Could you check a few things on this drawing? It's one solid part, dimensions in mm from its lowest x, y, z. Give positions to 0.01 mm unless a question says otherwise; leave off trailing zeros. Loops run counter-clockwise (first coordinate to the right, second up) from the corner with the lowest first, then second, coordinate; pieces in that order, holes last. Notation, with made-up numbers: M -29,69.25 L 10,69.25 A15 cw 10,76.25 Z; hole C 68.5,54 d1. An arc over 180 degrees is marked long. Answer as a JSON object with one key per item and string values.
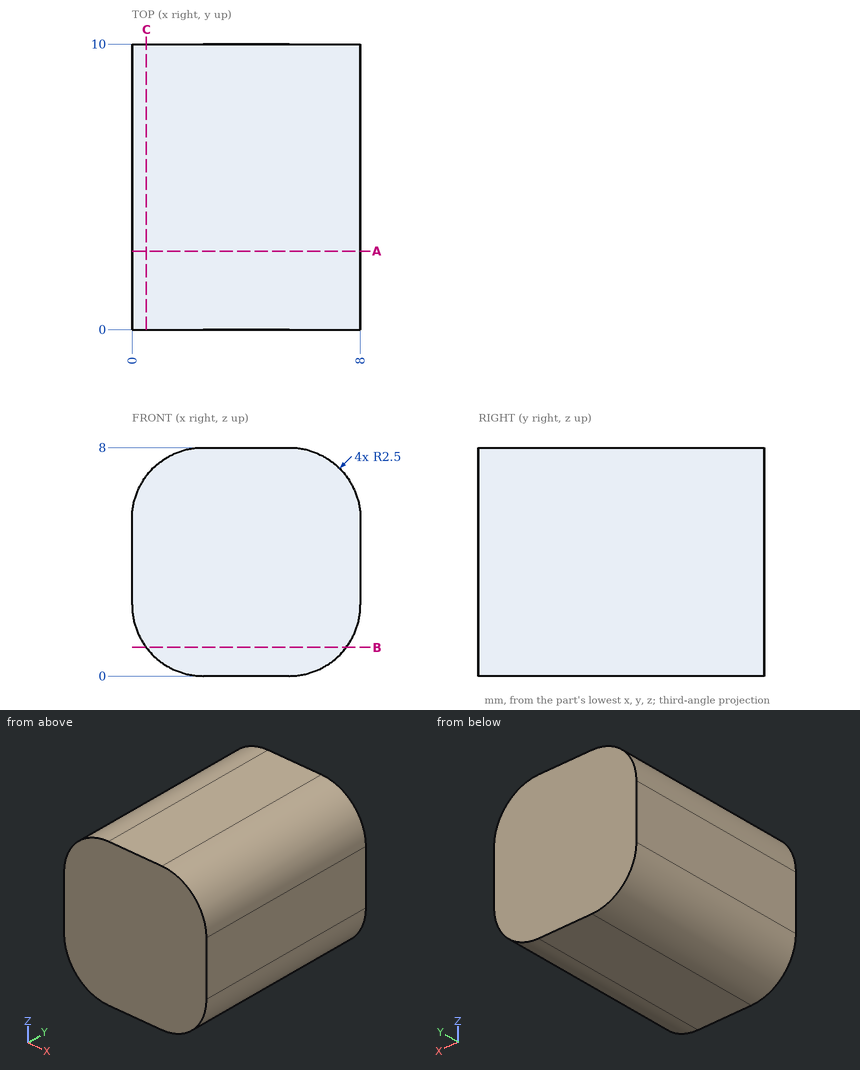
1) Suppose I cut it at C-C, the plane x = 0.5. Write out the boundary of the cut face in (y, z), and give its area (3 significant figures).
Answer list:
{"outline": "M 0,1 L 10,1 L 10,7 L 0,7 Z", "area": "60.0 mm^2"}
2) Will these pins go through, and if not, where does the flat tip stop? pin 1 Ø2 at (x, y) = (3, 1) entering from -Z; pin 2 Ø1.5 at (y, z) = (3, 6.5) entering from -X; pin 3 Ø2 at (y, z) = (6, 1) entering from +X.
Answer list:
{"pin 1": "z = 0", "pin 2": "x = 0.01", "pin 3": "x = 7.95"}
3) Suppose I cut it at B-B, the plane z = 1. Write out the boundary of the cut face in (x, y).
Answer list:
{"outline": "M 0.5,0 L 7.5,0 L 7.5,10 L 0.5,10 Z"}
4) Please list where these lines run through material, in increasing order: line 1 along X through (y, z) = (6.5, 6); line 2 along Z through (x, y) = (6.75, 0.75). Write a range as from..to.
Answer list:
{"line 1": "0.05..7.95", "line 2": "0.33..7.67"}
5) Suppose I cut it at A-A, the plane y = 2.75. Write out the boundary of the cut face in (x, z), and give its area (3 significant figures).
Answer list:
{"outline": "M 0,2.5 A2.5 ccw 2.5,0 L 5.5,0 A2.5 ccw 8,2.5 L 8,5.5 A2.5 ccw 5.5,8 L 2.5,8 A2.5 ccw 0,5.5 Z", "area": "58.6 mm^2"}
